Build history of the part. All positions in model axes, mm. Round coordinates to 2 decimals unless told otherwise and drop trailing zeros. Order: outer loops, then holes, each group sorted by start corner. A loop starts at its lowest first (then second) coordinate and runs counter-clockwise, first axis right, second up. Notation, with made-up numbers: (8, -6) -> (22, -6) arc R22 ccw to (22, 9) -> close; hole circle Ø5 at (24.5, 82). An arc over 180 degrees is marked (long way). Use a Markdown table: item, result. Add a question column.
Item 1: Pin check, flat tips, straight feed: pin 1 (2 mm diameter, centred on x = 22.85, y = 271.4, fed in from -Z); pin 2 (0.9 mm diameter, centred on x = 37.5, z = 1.5, fed in from -Y); pin 3 (1.5 mm diameter, centred on x = 28.5, z = 2, fed in from +Y); pin 4 (0.9 mm diameter, centred on x = 64, z = 1.5, fed in from -Y). Stop position of each tip, or through.
Item 2: Probe L1, parallel to X at y = 287.5, z = 2.35; L2, parallel to Y at x = 14.5, z = 2.3; L3, parallel to Y at x = 30, z = 1.7. List the from-to ranges inside material, lowest first.
Item 3: Two-plate mould, pull along X, no slides. Class faces 1 (the face through (65.296, 285, 1)), 2 (the face through (46, 298.852, 1)), 3 (the face through (36.69, 256.63, 1.48)), 4 (the face through (54.83, 256.62, 1.48)): released by +X, released by -X, zero draft, split by the parting line, or undercut.
Item 4: Slice it at B-B, the plane x = 46.5. State how many separate pieces and enclosed holes the cut face has, plus the area to 3 significant figures.
Item 5: Slice it at A-A, the plane x = 73. Give the cut face in (y, z), plus the area to 3 significant figures.
from build123d import *

# Parameters (mm, degrees)
MODEL_R                 = 1.25
MODEL_R_2               = 3.5
MODEL_R_3               = 1.5
MODEL_W                 = 9
MODEL_H                 = 3
MODEL_W_2               = 3
MODEL_H_2               = 9
SALIENTE_EXTRUIR1_DEPTH = 3


with BuildPart() as part:
    # Model → Saliente-Extruir1 (new body)
    with BuildSketch(Plane.XY):
        with BuildLine():
            Line((63.795544402, 295.852296768), (56.038185089, 295.852296768))
            ThreePointArc((56.038185089, 295.852296768), (54.890134792, 296.080658171), (53.916864745, 296.730976425))
            Line((53.916864745, 296.730976425), (52.674224058, 297.973617112))
            ThreePointArc((52.674224058, 297.973617112), (51.700954012, 298.623935366), (50.552903715, 298.852296768))
            Line((50.552903715, 298.852296768), (41.085229894, 298.852296768))
            ThreePointArc((41.085229894, 298.852296768), (39.937179597, 298.623935366), (38.96390955, 297.973617112))
            Line((38.96390955, 297.973617112), (37.721268863, 296.730976425))
            ThreePointArc((37.721268863, 296.730976425), (36.747998817, 296.080658171), (35.59994852, 295.852296768))
            Line((35.59994852, 295.852296768), (27.795544402, 295.852296768))
            ThreePointArc((27.795544402, 295.852296768), (8.295544402, 276.352296768), (27.795544402, 256.852296768))
            Line((27.795544402, 256.852296768), (35.552903715, 256.852296768))
            ThreePointArc((35.552903715, 256.852296768), (36.700954012, 256.623935366), (37.674224058, 255.973617112))
            Line((37.674224058, 255.973617112), (38.916864745, 254.730976425))
            ThreePointArc((38.916864745, 254.730976425), (39.890134792, 254.080658171), (41.038185089, 253.852296768))
            Line((41.038185089, 253.852296768), (50.50585891, 253.852296768))
            ThreePointArc((50.50585891, 253.852296768), (51.653909207, 254.080658171), (52.627179253, 254.730976425))
            Line((52.627179253, 254.730976425), (53.86981994, 255.973617112))
            ThreePointArc((53.86981994, 255.973617112), (54.843089987, 256.623935366), (55.991140284, 256.852296768))
            Line((55.991140284, 256.852296768), (63.795544402, 256.852296768))
            ThreePointArc((63.795544402, 256.852296768), (83.295544402, 276.352296768), (63.795544402, 295.852296768))
        make_face()
        with Locations((22.845796934, 281.302044237)):
            Circle(MODEL_R, mode=Mode.SUBTRACT)
        with Locations((22.845796934, 271.4025493)):
            Circle(MODEL_R, mode=Mode.SUBTRACT)
        with Locations((32.74529187, 271.4025493)):
            Circle(MODEL_R, mode=Mode.SUBTRACT)
        with Locations((32.74529187, 281.302044237)):
            Circle(MODEL_R, mode=Mode.SUBTRACT)
        with Locations((27.795544402, 276.352296768)):
            Circle(MODEL_R_2, mode=Mode.SUBTRACT)
        with Locations((18.795544402, 289.852296768)):
            Circle(MODEL_R_3, mode=Mode.SUBTRACT)
        with Locations((18.795544402, 262.852296768)):
            Circle(MODEL_R_3, mode=Mode.SUBTRACT)
        with Locations((36.795544402, 289.852296768)):
            Circle(MODEL_R_3, mode=Mode.SUBTRACT)
        with Locations((36.795544402, 262.852296768)):
            Circle(MODEL_R_3, mode=Mode.SUBTRACT)
        with Locations((14.295544402, 267.352296768)):
            Circle(MODEL_R_3, mode=Mode.SUBTRACT)
        with Locations((14.295544402, 285.352296768)):
            Circle(MODEL_R_3, mode=Mode.SUBTRACT)
        with Locations((30.977524917, 292.262199345)):
            Circle(MODEL_R_3, mode=Mode.SUBTRACT)
        with Locations((24.613563886, 260.442394192)):
            Circle(MODEL_R_3, mode=Mode.SUBTRACT)
        with Locations((30.977524917, 260.442394192)):
            Circle(MODEL_R_3, mode=Mode.SUBTRACT)
        with Locations((24.613563886, 292.262199345)):
            Circle(MODEL_R_3, mode=Mode.SUBTRACT)
        with Locations((11.885641825, 279.534277284)):
            Circle(MODEL_R_3, mode=Mode.SUBTRACT)
        with Locations((11.885641825, 273.170316253)):
            Circle(MODEL_R_3, mode=Mode.SUBTRACT)
        with Locations((58.845796933, 281.302044237)):
            Circle(MODEL_R, mode=Mode.SUBTRACT)
        with Locations((58.845796933, 271.4025493)):
            Circle(MODEL_R, mode=Mode.SUBTRACT)
        with Locations((68.74529187, 271.4025493)):
            Circle(MODEL_R, mode=Mode.SUBTRACT)
        with Locations((68.74529187, 281.302044237)):
            Circle(MODEL_R, mode=Mode.SUBTRACT)
        with Locations((54.795544402, 289.852296768)):
            Circle(MODEL_R_3, mode=Mode.SUBTRACT)
        with Locations((54.795544402, 262.852296768)):
            Circle(MODEL_R_3, mode=Mode.SUBTRACT)
        with Locations((72.795544402, 289.852296768)):
            Circle(MODEL_R_3, mode=Mode.SUBTRACT)
        with Locations((72.795544402, 262.852296768)):
            Circle(MODEL_R_3, mode=Mode.SUBTRACT)
        with Locations((77.295544402, 267.352296768)):
            Circle(MODEL_R_3, mode=Mode.SUBTRACT)
        with Locations((77.295544402, 285.352296768)):
            Circle(MODEL_R_3, mode=Mode.SUBTRACT)
        with Locations((66.977524917, 292.262199345)):
            Circle(MODEL_R_3, mode=Mode.SUBTRACT)
        with Locations((60.613563886, 260.442394192)):
            Circle(MODEL_R_3, mode=Mode.SUBTRACT)
        with Locations((66.977524917, 260.442394192)):
            Circle(MODEL_R_3, mode=Mode.SUBTRACT)
        with Locations((60.613563886, 292.262199345)):
            Circle(MODEL_R_3, mode=Mode.SUBTRACT)
        with Locations((79.705446979, 273.170316253)):
            Circle(MODEL_R_3, mode=Mode.SUBTRACT)
        with Locations((79.705446979, 279.534277284)):
            Circle(MODEL_R_3, mode=Mode.SUBTRACT)
        with Locations((63.795544402, 276.352296768)):
            Circle(MODEL_R_2, mode=Mode.SUBTRACT)
        with Locations((18.795544402, 285.352296768)):
            Circle(MODEL_R_3, mode=Mode.SUBTRACT)
        with Locations((18.795544402, 267.352296768)):
            Circle(MODEL_R_3, mode=Mode.SUBTRACT)
        with Locations((72.795544402, 285.352296768)):
            Circle(MODEL_R_3, mode=Mode.SUBTRACT)
        with Locations((72.795544402, 267.352296768)):
            Circle(MODEL_R_3, mode=Mode.SUBTRACT)
        with Locations((40.845796933, 281.302044237)):
            Circle(MODEL_R, mode=Mode.SUBTRACT)
        with Locations((40.845796933, 271.4025493)):
            Circle(MODEL_R, mode=Mode.SUBTRACT)
        with Locations((50.74529187, 271.4025493)):
            Circle(MODEL_R, mode=Mode.SUBTRACT)
        with Locations((50.74529187, 281.302044237)):
            Circle(MODEL_R, mode=Mode.SUBTRACT)
        with Locations((45.795544402, 276.352296768)):
            Circle(MODEL_R_2, mode=Mode.SUBTRACT)
        with Locations((41.295544402, 294.352296768)):
            Circle(MODEL_R_3, mode=Mode.SUBTRACT)
        with Locations((50.295544402, 294.352296768)):
            Circle(MODEL_R_3, mode=Mode.SUBTRACT)
        with Locations((45.795544402, 289.852296768)):
            Circle(MODEL_R_3, mode=Mode.SUBTRACT)
        with Locations((41.295544402, 258.352296768)):
            Circle(MODEL_R_3, mode=Mode.SUBTRACT)
        with Locations((50.295544402, 258.352296768)):
            Circle(MODEL_R_3, mode=Mode.SUBTRACT)
        with Locations((45.795544402, 262.852296768)):
            Circle(MODEL_R_3, mode=Mode.SUBTRACT)
        with Locations((36.795544402, 276.352296768)):
            Rectangle(MODEL_W, MODEL_H, mode=Mode.SUBTRACT)
        with Locations((27.795544402, 285.352296768)):
            Rectangle(MODEL_W_2, MODEL_H_2, mode=Mode.SUBTRACT)
        with Locations((18.795544402, 276.352296768)):
            Rectangle(MODEL_W, MODEL_H, mode=Mode.SUBTRACT)
        with Locations((27.795544402, 267.352296768)):
            Rectangle(MODEL_W_2, MODEL_H_2, mode=Mode.SUBTRACT)
        with Locations((72.795544402, 276.352296768)):
            Rectangle(MODEL_W, MODEL_H, mode=Mode.SUBTRACT)
        with Locations((63.795544402, 285.352296768)):
            Rectangle(MODEL_W_2, MODEL_H_2, mode=Mode.SUBTRACT)
        with Locations((54.795544402, 276.352296768)):
            Rectangle(MODEL_W, MODEL_H, mode=Mode.SUBTRACT)
        with Locations((63.795544402, 267.352296768)):
            Rectangle(MODEL_W_2, MODEL_H_2, mode=Mode.SUBTRACT)
        with Locations((36.795544402, 285.352296768)):
            Rectangle(MODEL_W_2, MODEL_H, mode=Mode.SUBTRACT)
        with Locations((45.795544402, 285.352296768)):
            Rectangle(MODEL_W_2, MODEL_H, mode=Mode.SUBTRACT)
        with Locations((54.795544402, 285.352296768)):
            Rectangle(MODEL_W_2, MODEL_H, mode=Mode.SUBTRACT)
        with Locations((36.795544402, 267.352296768)):
            Rectangle(MODEL_W_2, MODEL_H, mode=Mode.SUBTRACT)
        with Locations((45.795544402, 267.352296768)):
            Rectangle(MODEL_W_2, MODEL_H, mode=Mode.SUBTRACT)
        with Locations((54.795544402, 267.352296768)):
            Rectangle(MODEL_W_2, MODEL_H, mode=Mode.SUBTRACT)
        with Locations((45.795544402, 294.352296768)):
            Rectangle(MODEL_W_2, MODEL_H, mode=Mode.SUBTRACT)
        with Locations((45.795544402, 258.352296768)):
            Rectangle(MODEL_W_2, MODEL_H, mode=Mode.SUBTRACT)
    extrude(amount=SALIENTE_EXTRUIR1_DEPTH)


solid = part.part
Check sheet entries:
| question | item | result |
|---|---|---|
| 1 | pin 1 | through |
| 1 | pin 2 | y = 255.7 |
| 1 | pin 3 | y = 295.85 |
| 1 | pin 4 | y = 256.85 |
| 2 | L1 | 11.8 to 26.3, 29.3 to 62.3, 65.3 to 79.79 |
| 2 | L2 | 262.09 to 265.87, 268.84 to 274.85, 277.85 to 283.87, 286.84 to 290.62 |
| 2 | L3 | 256.85 to 259.3, 261.58 to 273.63, 279.07 to 291.12, 293.4 to 295.85 |
| 3 | face 1 | undercut |
| 3 | face 2 | zero draft |
| 3 | face 3 | released by -X |
| 3 | face 4 | released by +X |
| 4 | separate pieces | 8 |
| 4 | enclosed holes | 0 |
| 4 | area | 62.5 mm2 |
| 5 | outline | (259.16, 0) -> (261.37, 0) -> (261.37, 3) -> (259.16, 3) -> close; (264.34, 0) -> (265.87, 0) -> (265.87, 3) -> (264.34, 3) -> close; (268.84, 0) -> (274.85, 0) -> (274.85, 3) -> (268.84, 3) -> close; (277.85, 0) -> (283.87, 0) -> (283.87, 3) -> (277.85, 3) -> close; (286.84, 0) -> (288.37, 0) -> (288.37, 3) -> (286.84, 3) -> close; (291.34, 0) -> (293.54, 0) -> (293.54, 3) -> (291.34, 3) -> close |
| 5 | area | 58.5 mm2 |
